Input: part model. Units: mm. Frame: model coordinates. Round coordinates to 2 decimals unless told otherwise and drop trailing zeros. Order: outer loops, then holes, each group sorted by start corner. A loop starts at its lowest first (then second) coordinate and runs counter-clockwise, first axis right, second up. Notation, with made-up numbers: (11, 88) - (47, 88) arc R37 ccw to (47, 126) - close; hole circle Ø4 at (36, 75.25). An arc over 180 degrees is marked (long way). One line per item, written item: value. Start each with the question number.
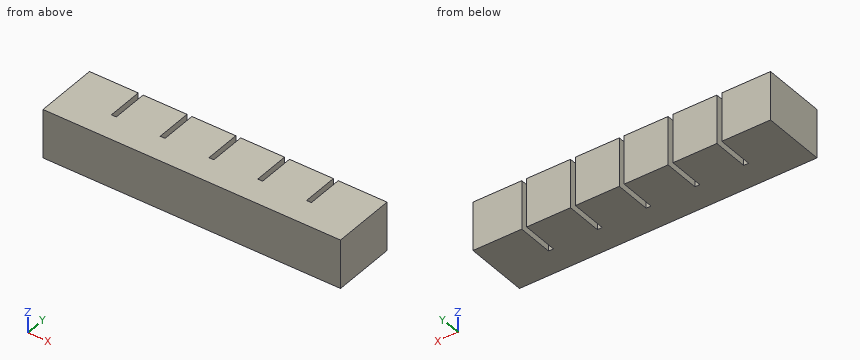
from build123d import *

# Parameters (mm, degrees)
SKETCH1_W           = 18
SKETCH1_H           = 20
BOSS_EXTRUDE1_DEPTH = 20
SKETCH2_W           = 10
SKETCH2_H           = 12
CUT_EXTRUDE1_DEPTH  = 16
SKETCH3_W           = 20
SKETCH3_H           = 5
BOSS_EXTRUDE2_DEPTH = 2
LPATTERN1_COUNT     = 6
LPATTERN1_PITCH     = 20
SKETCH4_W           = 20
SKETCH4_H           = 15
BOSS_EXTRUDE3_DEPTH = 2
SKETCH5_W           = 20
SKETCH5_H           = 20
BOSS_EXTRUDE4_DEPTH = 2
SKETCH6_W           = 110
SKETCH6_H           = 2
CUT_EXTRUDE2_DEPTH  = 2
SKETCH7_W           = 122
SKETCH7_H           = 20
BOSS_EXTRUDE5_DEPTH = 6


with BuildPart() as part:
    # Sketch1 → Boss-Extrude1 (new body)
    with BuildSketch(Plane.XY):
        with Locations((9, 10)):
            Rectangle(SKETCH1_W, SKETCH1_H)
    extrude(amount=BOSS_EXTRUDE1_DEPTH)

    # Sketch2 → Cut-Extrude1 (cut)
    with BuildSketch(Plane.XZ):
        with Locations((9, 10)):
            Rectangle(SKETCH2_W, SKETCH2_H)
    extrude(amount=-CUT_EXTRUDE1_DEPTH, mode=Mode.SUBTRACT)

    # Sketch3 → Boss-Extrude2 (add)
    with BuildSketch(Plane(origin=(18, 0, 0), x_dir=(0, 0, -1), z_dir=(1, 0, 0))):
        with Locations((-10, 2.5)):
            Rectangle(SKETCH3_W, SKETCH3_H)
    extrude(amount=BOSS_EXTRUDE2_DEPTH)


with BuildPart() as lpattern1_1:
    # LPattern1: pattern copy
    add(part.part.moved(Location(Vector(1, 0, 0) * (1 * LPATTERN1_PITCH))))


with BuildPart() as lpattern1_2:
    # LPattern1: pattern copy
    add(part.part.moved(Location(Vector(1, 0, 0) * (2 * LPATTERN1_PITCH))))


with BuildPart() as lpattern1_3:
    # LPattern1: pattern copy
    add(part.part.moved(Location(Vector(1, 0, 0) * (3 * LPATTERN1_PITCH))))


with BuildPart() as lpattern1_4:
    # LPattern1: pattern copy
    add(part.part.moved(Location(Vector(1, 0, 0) * (4 * LPATTERN1_PITCH))))


with BuildPart() as lpattern1_5:
    # LPattern1: pattern copy
    add(part.part.moved(Location(Vector(1, 0, 0) * (5 * LPATTERN1_PITCH))))

    # Sketch4 → Boss-Extrude3 (add)
    with BuildSketch(Plane(origin=(118, 0, 0), x_dir=(0, 0, -1), z_dir=(1, 0, 0))):
        with Locations((-10, 12.5)):
            Rectangle(SKETCH4_W, SKETCH4_H)
    extrude(amount=BOSS_EXTRUDE3_DEPTH)


with BuildPart() as part_1:
    add(part.part)

    # Sketch5 → Boss-Extrude4 (add)
    with BuildSketch(Plane.ZY):
        with Locations((10, 10)):
            Rectangle(SKETCH5_W, SKETCH5_H)
    extrude(amount=BOSS_EXTRUDE4_DEPTH)


with BuildPart() as lpattern1_1_1:
    add(lpattern1_1.part)

    # Combine1: union LPattern1_2, LPattern1_3, LPattern1_4, part, LPattern1_5
    add(lpattern1_2.part)
    add(lpattern1_3.part)
    add(lpattern1_4.part)
    add(part_1.part)
    add(lpattern1_5.part)

    # Sketch6 → Cut-Extrude2 (cut)
    with BuildSketch(Plane.XZ):
        with Locations((59, 10)):
            Rectangle(SKETCH6_W, SKETCH6_H)
    extrude(amount=-CUT_EXTRUDE2_DEPTH, mode=Mode.SUBTRACT)

    # Sketch7 → Boss-Extrude5 (add)
    with BuildSketch(Plane.XZ):
        with Locations((59, 10)):
            Rectangle(SKETCH7_W, SKETCH7_H)
    extrude(amount=BOSS_EXTRUDE5_DEPTH)


solid = lpattern1_1_1.part
1. Section C-C (y = 3.75). Return the cut outline in (x, z).
2. Section B-B (x = 47). Return the cut outline in (y, z).
3. Section A-A (y = 18). Return the cut outline in (x, z).
4. Line query: line 1 (X direction, y = 18.75, z = 15.25); line 2 (Y direction, x = 109, z = 8); line 3 (Z direction, x = 90.5, y = 4.5). Output: solid intervals per line, ascending. Write a range as from..to.
5. Section D-D (y = 8.25). State how many separate pieces and enclosed holes the cut face has, then the cut area to 3 significant figures.
Solved:
1. outline: (-2, 0) - (120, 0) - (120, 20) - (-2, 20) - close; hole (4, 4) - (14, 4) - (14, 16) - (4, 16) - close; hole (24, 4) - (34, 4) - (34, 16) - (24, 16) - close; hole (44, 4) - (54, 4) - (54, 16) - (44, 16) - close; hole (64, 4) - (74, 4) - (74, 16) - (64, 16) - close; hole (84, 4) - (94, 4) - (94, 16) - (84, 16) - close; hole (104, 4) - (114, 4) - (114, 16) - (104, 16) - close
2. outline: (-6, 0) - (20, 0) - (20, 20) - (-6, 20) - close; hole (0, 4) - (16, 4) - (16, 16) - (0, 16) - close
3. outline: (-2, 0) - (18, 0) - (18, 20) - (-2, 20) - close; (20, 0) - (38, 0) - (38, 20) - (20, 20) - close; (40, 0) - (58, 0) - (58, 20) - (40, 20) - close; (60, 0) - (78, 0) - (78, 20) - (60, 20) - close; (80, 0) - (98, 0) - (98, 20) - (80, 20) - close; (100, 0) - (120, 0) - (120, 20) - (100, 20) - close
4. line 1: x = -2..18, 20..38, 40..58, 60..78, 80..98, 100..120
4. line 2: y = -6..0, 16..20
4. line 3: z = 0..4, 16..20
5. separate pieces: 6
5. enclosed holes: 6
5. area: 1,520 mm²
